```python
from build123d import *

# Parameters (mm, degrees)
SKETCH1_W            = 5.409999999999997
SKETCH1_H            = 5.409999999999997
SKETCH1_W_2          = 4.549942703341507
SKETCH1_H_2          = 4.549942703341509
SKETCH1_W_3          = 0.4399999999999977
BOSS_EXTRUDE8_DEPTH  = 8.9
SKETCH2_W            = 0.24999999999999645
SKETCH2_H            = 1.5849393526398075
SKETCH2_W_2          = 0.25
CUT_EXTRUDE1_DEPTH   = 1
SKETCH3_W            = 2.0000000000000036
SKETCH3_H            = 0.1681942632906388
BOSS_EXTRUDE9_DEPTH  = 0.44
BOSS_EXTRUDE10_DEPTH = 2
SKETCH6_W            = 3.0119840570828487
SKETCH6_H            = 5.999459520470431
CUT_EXTRUDE2_DEPTH   = 10
SKETCH8_W            = 9
SKETCH8_H            = 17.909999999999997
BOSS_EXTRUDE11_DEPTH = 4.5
CHAMFER3_SIZE        = 3
CHAMFER3_SIZE2       = 4.2844440202263625
CHAMFER4_SIZE        = 1
CHAMFER4_SIZE2       = 4.331475874284207
SKETCH12_W           = 8.408099926910044
SKETCH12_H           = 4.631365679829861
CUT_EXTRUDE3_DEPTH   = 30
SHELL6_T             = -0.6
FILLET1_R            = 1.6
FILLET4_R            = 1.6


# Read off the part's stored shape, not the designer's step: Mirror5
with BuildPart() as part:
    # Sketch1 → Boss-Extrude8 (new body)
    # profile 1 of 10: a face of its own
    with BuildSketch(Plane(origin=(0, 0, 0), x_dir=(1, 0, 0), z_dir=(0, 1, 0))):
        with Locations((-39.80770033929644, 14.55082776302726)):
            Rectangle(SKETCH1_W, SKETCH1_H)
        with Locations((-39.79772898762569, 14.560799114698018)):
            Rectangle(SKETCH1_W_2, SKETCH1_H_2, mode=Mode.SUBTRACT)
    # profile 2 of 10: a face of its own
    with BuildSketch(Plane(origin=(0, 0, 0), x_dir=(1, 0, 0), z_dir=(0, 1, 0))):
        with Locations((-39.80770033929644, 14.560799114698018)):
            Rectangle(SKETCH1_W_3, SKETCH1_H_2)
    # profile 3 of 10: a face of its own
    with BuildSketch(Plane(origin=(0, 0, 0), x_dir=(1, 0, 0), z_dir=(0, 1, 0))):
        with BuildLine():
            ThreePointArc((-42.09264304263795, 17.25582776302726), (-42.302671690967195, 17.47082776302726), (-42.51270033929644, 17.25582776302726))
            Line((-42.51270033929644, 17.25582776302726), (-42.09264304263795, 17.25582776302726))
        make_face()
    # profile 4 of 10: a face of its own
    with BuildSketch(Plane(origin=(0, 0, 0), x_dir=(1, 0, 0), z_dir=(0, 1, 0))):
        with BuildLine():
            ThreePointArc((-42.51270033929644, 17.255827763027263), (-42.72270033929644, 17.035827763027264), (-42.51270033929644, 16.815827763027265))
            Line((-42.51270033929644, 16.815827763027265), (-42.51270033929644, 17.25582776302726))
        make_face()
    # profile 5 of 10: a face of its own
    with BuildSketch(Plane(origin=(0, 0, 0), x_dir=(1, 0, 0), z_dir=(0, 1, 0))):
        with BuildLine():
            ThreePointArc((-42.51270033929644, 12.285827763027262), (-42.722700339296445, 12.065827763027261), (-42.51270033929644, 11.84582776302726))
            Line((-42.51270033929644, 11.845827763027263), (-42.51270033929644, 12.285827763027262))
        make_face()
    # profile 6 of 10: a face of its own
    with BuildSketch(Plane(origin=(0, 0, 0), x_dir=(1, 0, 0), z_dir=(0, 1, 0))):
        with BuildLine():
            Line((-42.09264304263795, 11.845827763027263), (-42.51270033929644, 11.845827763027263))
            ThreePointArc((-42.51270033929644, 11.845827763027263), (-42.302671690967195, 11.630827763027263), (-42.09264304263795, 11.845827763027263))
        make_face()
    # profile 7 of 10: a face of its own
    with BuildSketch(Plane(origin=(0, 0, 0), x_dir=(1, 0, 0), z_dir=(0, 1, 0))):
        with BuildLine():
            Line((-37.10270033929644, 11.845827763027263), (-37.522757635954925, 11.845827763027263))
            ThreePointArc((-37.522757635954925, 11.845827763027263), (-37.31272898762568, 11.630827763027263), (-37.10270033929644, 11.845827763027263))
        make_face()
    # profile 8 of 10: a face of its own
    with BuildSketch(Plane(origin=(0, 0, 0), x_dir=(1, 0, 0), z_dir=(0, 1, 0))):
        with BuildLine():
            Line((-37.10270033929644, 12.285827763027264), (-37.10270033929644, 11.845827763027263))
            ThreePointArc((-37.10270033929644, 11.845827763027259), (-36.89270033929645, 12.065827763027261), (-37.10270033929644, 12.285827763027264))
        make_face()
    # profile 9 of 10: a face of its own
    with BuildSketch(Plane(origin=(0, 0, 0), x_dir=(1, 0, 0), z_dir=(0, 1, 0))):
        with BuildLine():
            ThreePointArc((-37.10270033929644, 17.25582776302726), (-37.31272898762568, 17.47082776302726), (-37.522757635954925, 17.25582776302726))
            Line((-37.522757635954925, 17.25582776302726), (-37.10270033929644, 17.25582776302726))
        make_face()
    # profile 10 of 10: a face of its own
    with BuildSketch(Plane(origin=(0, 0, 0), x_dir=(1, 0, 0), z_dir=(0, 1, 0))):
        with BuildLine():
            Line((-37.10270033929644, 17.25582776302726), (-37.10270033929644, 16.815827763027265))
            ThreePointArc((-37.10270033929644, 16.815827763027265), (-36.89270033929645, 17.035827763027264), (-37.10270033929644, 17.255827763027263))
        make_face()
    extrude(amount=BOSS_EXTRUDE8_DEPTH)

    # Sketch2 → Cut-Extrude1 (cut)
    with BuildSketch(Plane(origin=(-37.10270033929644, 0, 0), x_dir=(0, 0, -1), z_dir=(1, 0, 0))):
        Polygon((13.55082776302726, 7.315060647360192), (13.300827763027263, 7.315060647360192), (13.300827763027263, 3.9000000000000004), (13.550827763027263, 3.9), align=None)
        with Locations((13.42582776302726, 8.107530323680097)):
            Rectangle(SKETCH2_W, SKETCH2_H)
        with Locations((15.675827763027263, 8.107530323680097)):
            Rectangle(SKETCH2_W_2, SKETCH2_H)
        Polygon((15.800827763027263, 7.315060647360192), (15.550827763027263, 7.315060647360192), (15.550827763027264, 3.9000000000000004), (15.800827763027263, 3.9), align=None)
    extrude(amount=-CUT_EXTRUDE1_DEPTH, mode=Mode.SUBTRACT)

    # Sketch3 → Boss-Extrude9 (add)
    with BuildSketch(Plane(origin=(-37.10270033929644, 0, 0), x_dir=(0, 0, -1), z_dir=(1, 0, 0))):
        with Locations((14.55082776302726, 6.984097131645319)):
            Rectangle(SKETCH3_W, SKETCH3_H)
    extrude(amount=BOSS_EXTRUDE9_DEPTH)

    # Sketch5 → Boss-Extrude10 (add)
    with BuildSketch(Plane.XY.offset(-13.55082776302726)):
        Polygon((-36.662700339296435, 7.068194263290638), (-37.10270033929644, 8.9), (-37.10270033929644, 7.068194263290638), align=None)
    extrude(amount=-BOSS_EXTRUDE10_DEPTH)

    # Sketch6 → Cut-Extrude2 (cut)
    with BuildSketch(Plane(origin=(0, 8.9, 0), x_dir=(1, 0, 0), z_dir=(0, 1, 0))):
        with Locations((-41.31369236783786, 14.541370123902443)):
            Rectangle(SKETCH6_W, SKETCH6_H)
    extrude(amount=-CUT_EXTRUDE2_DEPTH, mode=Mode.SUBTRACT)

    # Sketch8 → Boss-Extrude11 (add)
    with BuildSketch(Plane.XZ):
        with Locations((-35.30770033929644, -13.80082776302726)):
            Rectangle(SKETCH8_W, SKETCH8_H)
    extrude(amount=-BOSS_EXTRUDE11_DEPTH)

    # Chamfer3
    chamfer3_edges = [part.edges().sort_by_distance(p)[0] for p in [
        (-30.80770033929644, 0, -13.80082776302726),
        (-35.30770033929644, 0, -4.845827763027263),
    ]]
    chamfer3_side = [part.faces().sort_by_distance(p)[0] for p in [
        (-35.30770033929644, 0, -13.80082776302726),
    ]]
    chamfer(chamfer3_edges, length=CHAMFER3_SIZE, length2=CHAMFER3_SIZE2, reference=chamfer3_side[0])

    # Chamfer4
    chamfer4_edges = [part.edges().sort_by_distance(p)[0] for p in [
        (-36.80770033929644, 0, -22.75582776302726),
    ]]
    chamfer4_side = [part.faces().sort_by_distance(p)[0] for p in [
        (-36.80770033929644, 0, -15.300827763027259),
    ]]
    chamfer(chamfer4_edges, length=CHAMFER4_SIZE, length2=CHAMFER4_SIZE2, reference=chamfer4_side[0])

    # Sketch12 → Cut-Extrude3 (cut)
    with BuildSketch(Plane.ZY.offset(39.80770033929644)):
        with Locations((-13.543811608056215, 6.81568283991493)):
            Rectangle(SKETCH12_W, SKETCH12_H)
    extrude(amount=-CUT_EXTRUDE3_DEPTH, mode=Mode.SUBTRACT)

    # Shell6
    shell6_openings = [part.faces().sort_by_distance(p)[0] for p in [
        (-39.807700339, 2.347603862, -14.251531758),
        (-35.307700339, 4.5, -13.800827763),
    ]]
    offset(amount=SHELL6_T, openings=shell6_openings, kind=Kind.INTERSECTION)

    # Mirror5: part across plane


with BuildPart() as part_1:
    add(part.part)
    add(part.part.mirror(Plane(origin=(-39.80770033929644, -1.1000000000000003, -17.541099884137658), x_dir=(0, 0, 1), z_dir=(1, 0, 0))))

    # Fillet1
    # the kernel refuses this fillet: 1.6 mm, written as the material it takes off along each edge
    with BuildSketch(Plane(origin=(-35.22184592572937, -2.0196092005073596, -9.259973349460195), x_dir=(0.2853788331334057, 0.40756321170586113, -0.867439421552548), z_dir=(0.4975428121645219, 0.7105647754616313, 0.4975428121645219))) as fillet1_piece_1:
        with BuildLine():
            CenterArc((FILLET1_R * 0.710564775462, FILLET1_R), FILLET1_R, 199.20747972534394, 70.79252027465611)
            Line((-FILLET1_R * 0.233768654558, FILLET1_R * 0.671010071663), (0, 0))
            Line((0, 0), (FILLET1_R * 0.710564775462, -5e-17))
        make_face()
    extrude(amount=11.714150079890267, mode=Mode.SUBTRACT)
    with BuildSketch(Plane(origin=(-44.39355475286351, -2.0196092005073587, -9.259973349460195), x_dir=(0.8674394215525482, 0.40756321170586235, 0.2853788331334039), z_dir=(-0.4975428121645219, 0.7105647754616313, 0.4975428121645219))) as fillet1_piece_2:
        with BuildLine():
            CenterArc((FILLET1_R * 0.710564775462, FILLET1_R), FILLET1_R, 199.20747972534403, 70.792520274656)
            Line((-FILLET1_R * 0.233768654558, FILLET1_R * 0.671010071663), (0, 0))
            Line((0, 0), (FILLET1_R * 0.710564775462, 1e-17))
        make_face()
    extrude(amount=11.714150079890267, mode=Mode.SUBTRACT)
    with BuildSketch(Plane(origin=(-43.82767365962377, -2.8277711558707384, -21.102985351354345), x_dir=(-0.10658333920242485, 0.1522167834338588, 0.9825833515002738), z_dir=(-0.5635866571713927, 0.8048851610657796, -0.1858223811990618))) as fillet1_piece_3:
        with BuildLine():
            CenterArc((FILLET1_R * 0.87831509781, FILLET1_R), FILLET1_R, 187.41334827823792, 82.58665172176217)
            Line((-FILLET1_R * 0.11332603197, FILLET1_R * 0.870973375896), (0, 0))
            Line((0, 0), (FILLET1_R * 0.87831509781, -2e-17))
        make_face()
    extrude(amount=12.349570861520077, mode=Mode.SUBTRACT)
    with BuildSketch(Plane(origin=(-35.78772701896911, -2.8277711558707392, -21.102985351354345), x_dir=(0.10658333920242458, 0.15221678343385903, 0.9825833515002738), z_dir=(0.5635866571713927, 0.8048851610657796, -0.1858223811990618))) as fillet1_piece_4:
        with BuildLine():
            CenterArc((FILLET1_R * 0.87831509781, -FILLET1_R), FILLET1_R, 89.99999999999993, 82.58665172176215)
            Line((-FILLET1_R * 0.11332603197, -FILLET1_R * 0.870973375896), (0, 0))
            Line((0, 0), (FILLET1_R * 0.87831509781, -1e-17))
        make_face()
    extrude(amount=12.349570861520073, mode=Mode.SUBTRACT)

    # Fillet4
    # the kernel refuses this fillet: 1.6 mm, written as the material it adds along each edge
    with BuildSketch(Plane(origin=(-49.62184592572936, 6.4932324940611, -4.031682176594339), x_dir=(0.867439421552548, 0.40756321170586235, 0.28537883313340373), z_dir=(0.4975428121645219, -0.7105647754616313, -0.4975428121645219))) as fillet4_piece_1_section:
        with BuildLine():
            CenterArc((FILLET4_R * 0.710564775462, -FILLET4_R), FILLET4_R, 89.99999999999997, 70.79252027465614)
            Line((-FILLET4_R * 0.233768654558, -FILLET4_R * 0.671010071663), (0, 0))
            Line((0, 0), (FILLET4_R * 0.710564775462, -1e-17))
        make_face()
    fillet4_piece_1 = extrude(amount=11.13598924099177, mode=Mode.PRIVATE)
    fillet4_piece_1 = split(fillet4_piece_1, bisect_by=Plane(origin=(-46.579824148031086, 4.5, -7.073703954292618), z_dir=(0, -1, 0)), keep=Keep.TOP, mode=Mode.PRIVATE)
    fillet4_piece_1 = split(fillet4_piece_1, bisect_by=Plane(origin=(-46.579824148031086, 0.6, -7.073703954292618), z_dir=(0, 1, 0)), keep=Keep.TOP, mode=Mode.PRIVATE)
    add(fillet4_piece_1)
    with BuildSketch(Plane(origin=(-29.993554752863513, 6.4932324940611, -4.031682176594337), x_dir=(-0.867439421552548, 0.40756321170586274, 0.28537883313340323), z_dir=(-0.4975428121645219, -0.7105647754616313, -0.4975428121645219))) as fillet4_piece_2_section:
        with BuildLine():
            CenterArc((FILLET4_R * 0.710564775462, FILLET4_R), FILLET4_R, 199.20747972534394, 70.79252027465606)
            Line((-FILLET4_R * 0.233768654558, FILLET4_R * 0.671010071663), (0, 0))
            Line((0, 0), (FILLET4_R * 0.710564775462, -6e-17))
        make_face()
    fillet4_piece_2 = extrude(amount=11.13598924099177, mode=Mode.PRIVATE)
    fillet4_piece_2 = split(fillet4_piece_2, bisect_by=Plane(origin=(-33.035576530561805, 4.5, -7.07370395429263), z_dir=(0, -1, 0)), keep=Keep.TOP, mode=Mode.PRIVATE)
    fillet4_piece_2 = split(fillet4_piece_2, bisect_by=Plane(origin=(-33.035576530561805, 0.6, -7.07370395429263), z_dir=(0, 1, 0)), keep=Keep.TOP, mode=Mode.PRIVATE)
    add(fillet4_piece_2)


solid = part_1.part
```
The model under review builds one solid part; all positions refer to its coordinate system, in mm. A direction names the side the tool comes from. Give positions to 0.01 mm unless a question says otherwise; leave off trailing zeros. Put each result on its own line as item: value.
(1) The part is to be moulded in two halves that separate along Z. For faces 3 (the flat face through (-39.691, 2.527, -21.723)), 4 (the flat face through (-47.329, 2.172, -13.842)), 5 (the flat face through (-39.705, 2.196, -22.263)), say which applies: pulls with the +Z half, pulls with the -Z half, needs draft (parallel to the pull), parting line crosses it, or undercut.
Results are:
face 3: undercut
face 4: needs draft
face 5: pulls with the -Z half
(2) Tool access review of faces 1 (the cylindrical face through (-33.149, 2.488, -7.207)), 2 (the cylindrical face through (-46.723, 2.019, -21.824)): name each direction out of +Z, -Z, +X, -X, +Y, -Y from which nothing blocks a thin tool from reaching the whole face with its end or side.
Results are:
face 1: +Y
face 2: -Z, -X, -Y
(3) To check wall thickness, follow probe 1 along Y at (x, z) = (-42.5, -16); probe 2 along X at (y, z) = (4.1, -11.25); probe 3 along Z at (x, y) = (-43.5, 1.45). State the ranges of each line that lie inside material, in increasing order. Write a range as from..to.
Results are:
probe 1: 0..0.6
probe 2: -48.68..-47.95, -31.67..-30.94
probe 3: -22.09..-21.47, -7.56..-6.83
(4) For pin 1 Ø1.5 at (y, z) = (3, -11) entering from +X; pin 2 Ø1 at (x, y) = (-40, 3) entering from -Z, all flat-tipped, find the tip position at first contact; note any pin that passes through.
Results are:
pin 1: x = -31.18
pin 2: z = -22.56
